Geometry check sheet. Reference: the model listing, model coordinates, mm. A direction names the side the tool comes from. Round coordinates to 2 decimals unless told otherwise and drop trailing zeros. Write each loop counter-clockwise with the first axis right and the second up, starting at its lowest first coordinate (ties: lowest second). Pieces come first, ordered by that corner, then holes. Notation, with made-up numbers: (-9.75, 76.5) - (10.25, 76.5) arc R23 cw to (10.25, 92.5) - close; hole circle Ø7 at (12, 53.25). An arc over 180 degrees is marked (long way). Return JSON: item names as keys, results as strings.
```python
from build123d import *

# Parameters (mm, degrees)
SKETCH_2_W           = 42
SKETCH_2_H           = 46
SKETCH_2_R           = 18.5
EXTRUDE_1_DEPTH      = 2
FILLET_1_R           = 5.5
SKETCH_3_R           = 1.6
CUT_EXTRUDE_1_DEPTH  = 32.208973069
SKETCH_4_R           = 4
SKETCH_4_R_2         = 2
EXTRUDE_2_DEPTH      = 2
SKETCH_7_R           = 1.5
EXTRUDE_4_DEPTH      = 2
EXTRUDE_5_DEPTH      = 7
EXTRUDE_5_DEPTH_BACK = 2
SKETCH_9_W           = 2
SKETCH_9_H           = 231
SKETCH_9_H_2         = 240
SKETCH_12_W          = 30
SKETCH_12_H          = 45
SKETCH_12_H_2        = 80
CUT_EXTRUDE_4_DEPTH  = 222.592303341
EXTRUDE_6_DEPTH      = 2
EXTRUDE_7_DEPTH      = 2
FILLET_2_R           = 3
SKETCH_15_R          = 1.5
CUT_EXTRUDE_5_DEPTH  = 222.592303341


with BuildPart() as part:
    # 草图2 → 凸台-拉伸1 (new body)
    with BuildSketch(Plane(origin=(0, 0, 0), x_dir=(1, 0, 0), z_dir=(0, 1, 0))):
        Rectangle(SKETCH_2_W, SKETCH_2_H)
        with Locations(Location((0, 0, 0), (0, 0, 270))):
            Circle(SKETCH_2_R, mode=Mode.SUBTRACT)
    extrude(amount=EXTRUDE_1_DEPTH)

    # 圆角1
    fillet_1_edges = [part.edges().sort_by_distance(p)[0] for p in [
        (-21, 1, -23),
    ]]
    fillet(fillet_1_edges, radius=FILLET_1_R)

    # 草图3 → 切除-拉伸1 (cut, through all)
    with BuildSketch(Plane(origin=(0, 2, 0), x_dir=(1, 0, 0), z_dir=(0, 1, 0))):
        with Locations(Location((-15.5, 15.5, 0), (0, 0, 270))):
            Circle(SKETCH_3_R)
        with Locations(Location((15.5, 15.5, 0), (0, 0, 270))):
            Circle(SKETCH_3_R)
        with Locations(Location((-15.5, -15.5, 0), (0, 0, 270))):
            Circle(SKETCH_3_R)
        with Locations(Location((15.5, -15.5, 0), (0, 0, 270))):
            Circle(SKETCH_3_R)
    extrude(amount=-CUT_EXTRUDE_1_DEPTH, mode=Mode.SUBTRACT)

    # 草图4 → 凸台-拉伸2 (add)
    with BuildSketch(Plane(origin=(0, 2, 0), x_dir=(1, 0, 0), z_dir=(0, 1, 0))):
        Polygon((-21, -23), (21, -23), (21, -176), (21, -217), (-21, -217), (-21, -176), align=None)
        with Locations(Location((0, -195, 0), (0, 0, 270))):
            Circle(SKETCH_4_R, mode=Mode.SUBTRACT)
        with Locations(Location((10.253048327, -184.746951673, 0), (0, 0, 270))):
            Circle(SKETCH_4_R_2, mode=Mode.SUBTRACT)
        with Locations(Location((-10.253048327, -184.746951673, 0), (0, 0, 270))):
            Circle(SKETCH_4_R_2, mode=Mode.SUBTRACT)
        with Locations(Location((10.253048327, -205.253048327, 0), (0, 0, 270))):
            Circle(SKETCH_4_R_2, mode=Mode.SUBTRACT)
        with Locations(Location((-10.253048327, -205.253048327, 0), (0, 0, 270))):
            Circle(SKETCH_4_R_2, mode=Mode.SUBTRACT)
    extrude(amount=-EXTRUDE_2_DEPTH)

    # 草图7 → 凸台-拉伸4 (add)
    with BuildSketch(Plane(origin=(0, 2, 0), x_dir=(1, 0, 0), z_dir=(0, 1, 0))):
        Polygon((-15.5, 23), (-21, 17), (-21, 27), (-41.33, 27), (-44.33, 27), (-44.33, 33), (-41.33, 33), (-15.5, 33), align=None)
        with Locations(Location((-41.33, 30, 0), (0, 0, 270))):
            Circle(SKETCH_7_R, mode=Mode.SUBTRACT)
        with Locations(Location((-22, 30, 0), (0, 0, 270))):
            Circle(SKETCH_7_R, mode=Mode.SUBTRACT)
    extrude(amount=-EXTRUDE_4_DEPTH)

    # 草图9 → 凸台-拉伸5 (add, two sides: drawn at the far end of the back side and taken through both)
    with BuildSketch(Plane(origin=(0, 2, 0), x_dir=(1, 0, 0), z_dir=(0, 1, 0)).offset(-EXTRUDE_5_DEPTH_BACK)):
        with Locations((-22, -101.5)):
            Rectangle(SKETCH_9_W, SKETCH_9_H)
        with Locations((22, -97)):
            Rectangle(SKETCH_9_W, SKETCH_9_H_2)
    extrude(amount=EXTRUDE_5_DEPTH + EXTRUDE_5_DEPTH_BACK)

    # 草图12 → 切除-拉伸4 (cut, through all)
    with BuildSketch(Plane(origin=(0, 2, 0), x_dir=(1, 0, 0), z_dir=(0, 1, 0))):
        with Locations((0, -45)):
            Rectangle(SKETCH_12_W, SKETCH_12_H)
        with Locations((0, -130)):
            Rectangle(SKETCH_12_W, SKETCH_12_H_2)
    extrude(amount=-CUT_EXTRUDE_4_DEPTH, mode=Mode.SUBTRACT)

    # 草图13 → 凸台-拉伸6 (add)
    with BuildSketch(Plane(origin=(0, 2, 0), x_dir=(1, 0, 0), z_dir=(0, 1, 0))):
        Polygon((-17.080125736, -23.886750491), (12.919874264, -68.886750491), (17.080125736, -66.113249509), (-12.919874264, -21.113249509), align=None)
        Polygon((-17.340822944, -90.877808604), (12.659177056, -170.877808604), (17.340822944, -169.122191396), (-12.659177056, -89.122191396), align=None)
    extrude(amount=-EXTRUDE_6_DEPTH)

    # 草图14 → 凸台-拉伸7 (add)
    with BuildSketch(Plane(origin=(0, 2, 0), x_dir=(1, 0, 0), z_dir=(0, 1, 0))):
        Polygon((-17.080125736, -66.113249509), (12.919874264, -21.113249509), (17.080125736, -23.886750491), (-12.919874264, -68.886750491), align=None)
        Polygon((-17.340822944, -169.122191396), (12.659177056, -89.122191396), (17.340822944, -90.877808604), (-12.659177056, -170.877808604), align=None)
    extrude(amount=-EXTRUDE_7_DEPTH)

    # 圆角2
    fillet_2_edges = [part.edges().sort_by_distance(p)[0] for p in [
        (-15.5, 1, -23),
        (-15.5, 1, -33),
        (-21, 1, -27),
        (-44.33, 1, -27),
        (-44.33, 1, -33),
    ]]
    fillet(fillet_2_edges, radius=FILLET_2_R - 0.0001)  # a hair under: the kernel refuses the full size

    # 草图15 → 切除-拉伸5 (cut, through all)
    with BuildSketch(Plane(origin=(0, 2, 0), x_dir=(1, 0, 0), z_dir=(0, 1, 0))):
        with Locations(Location((0, -78.75, 0), (0, 0, 270))):
            Circle(SKETCH_15_R)
        with Locations(Location((12, -78.75, 0), (0, 0, 270))):
            Circle(SKETCH_15_R)
        with Locations(Location((-12, -78.75, 0), (0, 0, 270))):
            Circle(SKETCH_15_R)
    extrude(amount=-CUT_EXTRUDE_5_DEPTH, mode=Mode.SUBTRACT)


solid = part.part
```
(1) Section check A-A, the plane y = 5. Enter the section's corners in (x, z).
Response values:
{"outline": "(-23, -14) - (-21, -14) - (-21, 217) - (-23, 217) - close; (21, -23) - (23, -23) - (23, 217) - (21, 217) - close"}
(2) Access from +Z, -Z, +X, -X, +Y, -Y to the whole of each face (thin tool, end or side, straight path). Record for faces 1 (the face through (4, 0, 118)), 2 (the face through (-23, 4, 103)), 3 (the face through (6.08, 1.01, 106.67)), 4 (the face through (21, 5, 99)), 5 (the face through (23, 4, 99)).
Response values:
{"face 1": "+Z, -Z, +X, -X, -Y", "face 2": "+Z, -X, +Y, -Y", "face 3": "+Y, -Y", "face 4": "+Z, -Z, +Y", "face 5": "+Z, -Z, +X, +Y, -Y"}
(3) Gauge pin test, flat ends, axial feed: pin 1 (1 mm diameter, centred on y = 5.5, z = 102, fed in from -X); pin 2 (5 mm diameter, centred on x = -13, z = 96, fed in from +Y); pin 3 (3 mm diameter, centred on x = -23.5, y = 2.5, fed in from +Z); pin 4 (1.6 mm diameter, centred on y = 1, z = -20, fed in from -X). Record the tip position at first contact, or that the pin passes through.
Response values:
{"pin 1": "stops at x = -23", "pin 2": "stops at y = 2", "pin 3": "stops at z = 217", "pin 4": "stops at x = -21"}
(4) Section check D-D, the plane x = -34. Enter the section's corners in (y, z), plus the area to 3 significant figures.
Response values:
{"outline": "(0, -33) - (2, -33) - (2, -27) - (0, -27) - close", "area": "12.0 mm^2"}
(5) Material ranges on line 1 along X through (y, z) = (0.6, -30); line 2 along X through (y, z) = (4.75, 123); line 3 along X through (y, z) = (1.25, 58), recorded low to high. Write a range as [from, to].
Response values:
{"line 1": "x = [-44.33, -42.83], [-39.83, -23.5], [-20.5, -15.5]", "line 2": "x = [-23, -21], [21, 23]", "line 3": "x = [-23, -15], [-11.67, -5.66], [5.66, 11.67], [15, 23]"}
(6) Release check for a two-part mould opening along Z. For faces 6 (the face through (5.914, 1.014, 31.622)), 7 (the face through (-11.019, 1.014, 186.594)), 8 (the face through (0, 1, 217)), 9 (the face through (-4, 2, 118)) record: pulls with the +Z half, pulls with the -Z half, needs draft (parallel to the pull), parting line crosses it, or undercut.
Response values:
{"face 6": "undercut", "face 7": "undercut", "face 8": "pulls with the +Z half", "face 9": "needs draft"}
(7) Section check C-C, the plane z = 9. Enter the section's corners in (x, y).
Response values:
{"outline": "(-23, 0) - (-16.16, 0) - (-16.16, 2) - (-21, 2) - (-21, 9) - (-23, 9) - close; (16.16, 0) - (23, 0) - (23, 9) - (21, 9) - (21, 2) - (16.16, 2) - close"}
(8) Section check B-B, the plane z = 57. Enter the section's corners in (x, y).
Response values:
{"outline": "(-23, 0) - (-15, 0) - (-15, 2) - (-21, 2) - (-21, 9) - (-23, 9) - close; (-11, 0) - (-5, 0) - (-5, 2) - (-11, 2) - close; (5, 0) - (11, 0) - (11, 2) - (5, 2) - close; (15, 0) - (23, 0) - (23, 9) - (21, 9) - (21, 2) - (15, 2) - close"}
